The listing builds one solid part. Answer for the finished solid, in the listing's coordinates (mm). A direction names the side the tool comes from. Coordinates: 2 decimals unless noted, no trailing zeros. Order: outer loops, then holes, each group sorted by start corner. A loop starts at its lowest first (then second) coordinate and runs counter-clockwise, first axis right, second up.
```python
from build123d import *

# Parameters (mm, degrees)
SKETCH1_W             = 57
SKETCH1_H             = 41.5
BOSS_EXTRUDE1_DEPTH   = 1
SKETCH2_W             = 57
SKETCH2_H             = 38
BOSS_EXTRUDE2_DEPTH   = 6
F_1_0MM_DOWEL_HOLE1_D = 1.6


with BuildPart() as part:
    # Sketch1 → Boss-Extrude1 (new body)
    with BuildSketch(Plane.XY):
        with Locations((28.5, 20.75)):
            Rectangle(SKETCH1_W, SKETCH1_H)
    extrude(amount=BOSS_EXTRUDE1_DEPTH)

    # Sketch2 → Boss-Extrude2 (add)
    with BuildSketch(Plane.XY.offset(1)):
        with Locations((28.5, 22.5)):
            Rectangle(SKETCH2_W, SKETCH2_H)
    extrude(amount=BOSS_EXTRUDE2_DEPTH)

    # Ø1.0mm Dowel Hole1 (through all)
    with Locations(Plane(origin=(10, 1.5, 1), x_dir=(1, 0, 0), z_dir=(0, 0, 1))):
        with Locations((0, 0)):
            Hole(F_1_0MM_DOWEL_HOLE1_D / 2)


solid = part.part
```
(1) Find section D-D (z = 3). Write down the section's boundary in (x, y), and give its area (3 significant figures).
(2) Find section A-A (x = 10). Write down the section's boundary in (y, z), and give its area (3 significant figures).
(3) Find section B-B (y = 1.5). Write down the section's boundary in (x, z).
(4) Each of these flat-tipped pins is pushed along its axis until it touches: pin 1 Ø1 at (x, z) = (9, 3.5) entering from -Y; pin 2 Ø1.8 at (x, y) = (33.5, 2.5) entering from +Z. Where does it stop, or does it pass through?
(5) Find section C-C (x = 19). Write down the section's boundary in (y, z), and give its area (4 significant figures).
(6) The mould has two halves that part along X. Classify faces 1 (the face through (28, 41.5, 3)), 2 (the face through (10.63, 1.01, 0.49)), 3 (the face through (57, 20, 3)): released by +X, released by -X, zero draft, split by the parting line, or undercut.
(7) For faces 4 (the face through (28, 2, 1)), 5 (the face through (0, 20, 3)), determine the directions among +Z, -Z, +X, -X, +Y, -Y from which every point of the face is accessible in a straight line to the end or side of a thin tool.
(8) Consider line 1 (Y direction, x = 10, z = 0.35); line 2 (Y direction, x = 35, z = 5.75); line 3 (Z direction, x = 15, y = 2). Determine where each line is inside the solid, lowest interval first.
Findings below:
1. outline: (0, 3.5) - (57, 3.5) - (57, 41.5) - (0, 41.5) - close
1. area: 2,170 mm2
2. outline: (0, 0) - (0.7, 0) - (0.7, 1) - (0, 1) - close; (2.3, 0) - (41.5, 0) - (41.5, 7) - (3.5, 7) - (3.5, 1) - (2.3, 1) - close
2. area: 268 mm2
3. outline: (0, 0) - (9.2, 0) - (9.2, 1) - (0, 1) - close; (10.8, 0) - (57, 0) - (57, 1) - (10.8, 1) - close
4. pin 1: stops at y = 3.5
4. pin 2: stops at z = 1
5. outline: (0, 0) - (41.5, 0) - (41.5, 7) - (3.5, 7) - (3.5, 1) - (0, 1) - close
5. area: 269.5 mm2
6. face 1: zero draft
6. face 2: undercut
6. face 3: released by +X
7. face 4: +Z, +X, -X, -Y
7. face 5: +Z, -Z, -X, +Y, -Y
8. line 1: y = 0 to 0.7, 2.3 to 41.5
8. line 2: y = 3.5 to 41.5
8. line 3: z = 0 to 1
